Verification items for the finished model (mm, model axes). A direction names the side the tool comes from. Coordinates: 2 decimals unless noted, no trailing zeros. Write each loop counter-clockwise with the first axis right and the second up, starting at its lowest first coordinate (ties: lowest second). Pieces come first, ordered by that corner, then holes.
Autodesk Inventor part; units mm, degrees
ref_plane "YZ Plane" through (0, 0, 0) normal (1, 0, 0) x (0, 1, 0)
ref_plane "XZ Plane" through (0, 0, 0) normal (0, 1, 0) x (-1, 0, 0)
ref_plane "XY Plane" through (0, 0, 0) normal (0, 0, 1) x (1, 0, 0)
sketch "Sketch1" plane through (0, 0, 0) normal (0, 0, 1) x (1, 0, 0)
  circle A0 centre (0, 0) radius 4
  dimension "d0" = 8
extrude "Extrusion1" add sketch "Sketch1" along normal blind 160
sketch "Sketch2" plane through (0, 0, 160) normal (0, 0, 1) x (1, 0, 0)
  line L0 (-2.5278, 3.1) -> (2.5278, 3.1)
  line L1 (2.5278, -3.1) -> (-2.5278, -3.1)
  arc A0 (-2.5278, 3.1) -> (-2.5278, -3.1) centre (0, 0) ccw
  arc A1 (2.5278, -3.1) -> (2.5278, 3.1) centre (0, 0) ccw
  line L2 (-2.5278, 3.1) -> (3.1486, 3.1)
  line L3 (3.1486, 3.1) -> (3.1486, 5.5336)
  line L4 (3.1486, 5.5336) -> (-2.5278, 5.5336)
  line L5 (-2.5278, 5.5336) -> (-2.5278, 3.1)
  line L6 (2.5278, -3.1) -> (-2.7681, -3.1)
  line L7 (-2.7681, -3.1) -> (-2.7681, -5.0994)
  line L8 (-2.7681, -5.0994) -> (2.5278, -5.0994)
  line L9 (2.5278, -5.0994) -> (2.5278, -3.1)
  dimension "d3" = 3.1
extrude "Extrusion2" cut sketch "Sketch2" against normal blind 30 contours L5 L4 L3 L2 L0 | L1 L9 L8 L7 L6
properties part number "oś napędowa"
1. Sectioned sample at C-C, the plane y = -1.5. Record the boundary of the cut face in (x, z).
2. Material ranges on L1, parallel to Y at x = 2.5, z = 108; L2, parallel to Y at x = -0.5, z = 30, recorded low to high.
3. Tool access check on faces 1 (the flat face through (0, 3.1, 145)), 2 (the flat face through (0, -3.1, 145)), 3 (the cylindrical face through (-4, 0, 79)). Record the directions out of +Z, -Z, +X, -X, +Y, -Y that give a thin tool (end or side, any length) a straight path to the whole face; none if there is none.
4. Sectioned sample at A-A, the plane x = 0. Record the boundary of the cut face in (y, z).
5. Gauge pin test, flat ends, axial feed: P1, Ø1.5, axis at x = 0, z = 149, coming from the -Y side; P2, Ø1, axis at x = 1, z = 101.5, coming from the -Y side; P3, Ø0.5, axis at x = -1, y = -3.5, coming from the +Z side; P4, Ø1, axis at x = 0, y = 3.5, coming from the +Z side. Record the tip position at first contact, or that the pin passes through.
6. Sectioned sample at D-D, the plane z = 114.5. Record the boundary of the cut face in (x, y), and give its area (3 significant figures).
Outcome:
1. outline: (-3.71, 0) - (3.71, 0) - (3.71, 160) - (-3.71, 160) - close
2. L1: y = -3.12 to 3.12
2. L2: y = -3.97 to 3.97
3. face 1: +Z, +X, -X, +Y
3. face 2: +Z, +X, -X, -Y
3. face 3: +Z, -Z
4. outline: (-4, 0) - (4, 0) - (4, 130) - (3.1, 130) - (3.1, 160) - (-3.1, 160) - (-3.1, 130) - (-4, 130) - close
5. P1: stops at y = -3.1
5. P2: stops at y = -3.97
5. P3: stops at z = 130
5. P4: stops at z = 160
6. outline: circle Ø8 at (0, 0)
6. area: 50.3 mm2
